Input: part model. Units: mm. Frame: model coordinates. A direction names the side the tool comes from. Coordinates: 2 decimals unless noted, no trailing zeros. Loops run counter-clockwise (first coordinate to the right, second up) from the corner with the lowest first, then second, coordinate; pieces in that order, holes last.
(1) Contact query for flat-ended pins moving along their axis: P1, Ø8, axis at x = 3, y = 16.5, coming from the -Z side; P2, Ø2, axis at y = 17, z = 42, coming from the +X side; P3, Ø1, axis at x = 3.5, y = 28.5, coming from the +Z side. Output: stop coordinate, or through.
(2) Set-up query: faces 1 (the face through (11, 20, 68)), 2 (the face through (21, 20, 69)). Return all of +Z, -Z, +X, -X, +Y, -Y with unobstructed straight access to the full face (end or side cutting, diameter ignored); none if empty.
(3) Section C-C, the plane z = 16. Return loops of the section in (x, y), then the cut area to 3 significant figures.
(4) Section D-D, the plane x = 14.75. Return loops of the section in (y, z), then the cut area to 3 significant figures.
(5) Mould query, pull axis Z, two halves, no side actions, for faces 3 (the face through (1, 20, 35)), 4 (the face through (10.35, 20.28, -5.07)), 5 (the face through (0.3, 40, 34.8)), 6 (the face through (11, 20, 2)). Classes: released by +Z, released by -Z, zero draft, split by the parting line, or undercut.
(6) Section B-B, the plane y = 18. Return loops of the section in (x, z), then the cut area to 3 significant figures.
(7) Line query: L1, parallel to X at y = 37.5, z = 15.5; L2, parallel to Z at x = 12.25, y = 2.5; L3, parallel to Z at x = 16, y = 28. Output: solid intervals per line, ascending.
(8) Section A-A, the plane x = 5.25. Return loops of the section in (y, z).
Autodesk Inventor part; units mm, degrees
ref_plane "YZ Plane" through (0, 0, 0) normal (1, 0, 0) x (0, 1, 0)
ref_plane "XZ Plane" through (0, 0, 0) normal (0, 1, 0) x (-1, 0, 0)
ref_plane "XY Plane" through (0, 0, 0) normal (0, 0, 1) x (1, 0, 0)
sketch "Sketch1" plane through (0, 0, 0) normal (1, 0, 0) x (0, 1, 0)
  line L0 (0, 0) -> (40, 0)
  line L1 (40, 0) -> (40, 70)
  line L2 (40, 70) -> (0, 70)
  line L3 (0, 70) -> (0, 0)
  dimension "d0" = 40
  dimension "d1" = 70
extrude "Extrusion1" add sketch "Sketch1" along normal blind 1
sketch "Sketch2" plane through (1, 0, 0) normal (1, 0, 0) x (0, 0, -1)
  line L0 (-70, 40) -> (-70, 0)
  line L1 (-70, 0) -> (0, 0)
  line L2 (-70, 40) -> (-68, 40)
  line L3 (-68, 40) -> (-68, 0)
  line L4 (-68, 0) -> (-70, 0)
  line L5 (-70, 0) -> (-70, 40)
  line L6 (0, 0) -> (0, 40)
  line L7 (0, 40) -> (-2, 40)
  line L8 (-2, 40) -> (-2, 0)
  line L9 (-2, 0) -> (0, 0)
  line L10 (0, 0) -> (0, 40)
  dimension "d4" = 2
  dimension "d5" = 2
extrude "Extrusion2" add sketch "Sketch2" along normal blind 20
sketch "Sketch4" plane through (0, 40, 70) normal (0, 1, 0) x (1, 0, 0)
  line L0 (0, 70) -> (0, 80)
  line L1 (21, 68) -> (21, 70)
  line L2 (0, 80) -> (21, 70)
  line L3 (0, 70) -> (0, 0)
  line L4 (0, 0) -> (0, -10)
  line L5 (0, 0) -> (21, 0)
  line L6 (0, -10) -> (21, 0)
  line L7 (0, 70) -> (21, 70)
  line L8 (1, 68) -> (21, 68)
  dimension "d8" = 10
  dimension "d9" = 10
extrude "Extrusion3" add sketch "Sketch4" against normal blind 40
properties part number "MAN_BASIS_GRIPPER" material "ABS Plastic"
Report:
1. P1: stops at z = -10
1. P2: stops at x = 1
1. P3: stops at z = 78.57
2. face 1: +X, +Y, -Y
2. face 2: +Z, -Z, +X, +Y, -Y
3. outline: (0, 0) - (1, 0) - (1, 40) - (0, 40) - close
3. area: 40.0 mm2
4. outline: (0, -2.98) - (40, -2.98) - (40, 2) - (0, 2) - close; (0, 68) - (40, 68) - (40, 72.98) - (0, 72.98) - close
4. area: 398 mm2
5. face 3: undercut
5. face 4: released by -Z
5. face 5: zero draft
5. face 6: undercut
6. outline: (0, -10) - (21, 0) - (21, 2) - (1, 2) - (1, 68) - (21, 68) - (21, 70) - (0, 80) - close
6. area: 360 mm2
7. L1: x = 0 to 1
7. L2: z = -4.17 to 2, 68 to 74.17
7. L3: z = -2.38 to 2, 68 to 72.38
8. outline: (0, -7.5) - (40, -7.5) - (40, 2) - (0, 2) - close; (0, 68) - (40, 68) - (40, 77.5) - (0, 77.5) - close
